from build123d import *

# Parameters (mm, degrees)
SALIENTE_EXTRUIR1_DEPTH = 49
CORTAR_EXTRUIR1_DEPTH   = 70.738798384
SALIENTE_EXTRUIR3_DEPTH = 10
CROQUIS8_W              = 12
CROQUIS8_H              = 10
CORTAR_EXTRUIR2_DEPTH   = 6.5
CROQUIS9_W              = 20
CROQUIS9_H              = 12
SALIENTE_EXTRUIR4_DEPTH = 1.5
CROQUIS10_W             = 49
CROQUIS10_H             = 45
CORTAR_EXTRUIR6_DEPTH   = 16
CROQUIS13_W             = 2
CROQUIS13_H             = 10
CORTAR_EXTRUIR7_DEPTH   = 64.131209746


with BuildPart() as part:
    # Croquis1 → Saliente-Extruir1 (new body)
    with BuildSketch(Plane.XY):
        Polygon((-3.5, 49.5), (-3.5, 0), (0, 0), (0, 41.994225778), align=None)
    extrude(amount=SALIENTE_EXTRUIR1_DEPTH)

    # Croquis2 → Cortar-Extruir1 (cut, through all)
    with BuildSketch(Plane(origin=(0, 0, 0), x_dir=(0, 0, -1), z_dir=(1, 0, 0))):
        Polygon((-49, 0), (0, 0), (0, 28.994225778), (-14.5, 28.994225778), (-14.5, 4.5), (-34.5, 4.5), (-34.5, 28.994225778), (-49, 28.994225778), align=None)
    extrude(amount=-CORTAR_EXTRUIR1_DEPTH, mode=Mode.SUBTRACT)

    # Croquis4 → Saliente-Extruir3 (add)
    with BuildSketch(Plane.XZ.offset(-28.994225778)):
        Polygon((0, 49), (20.5, 49), (20.5, 0), (0, 0), (0, 1.5), (12.5, 1.5), (12.5, 47.5), (0, 47.5), align=None)
    extrude(amount=-SALIENTE_EXTRUIR3_DEPTH)

    # Croquis8 → Cortar-Extruir2 (cut)
    with BuildSketch(Plane(origin=(20.5, 0, 0), x_dir=(0, 0, -1), z_dir=(1, 0, 0))):
        with Locations((-24.5, 33.994225778)):
            Rectangle(CROQUIS8_W, CROQUIS8_H)
        Polygon((-48, 38.994225778), (-44.360297657, 28.994225778), (-31.590164388, 28.994225778), (-35.22986673, 38.994225778), align=None)
        Polygon((-17.409835612, 28.994225778), (-4.639702343, 28.994225778), (-1, 38.994225778), (-13.77013327, 38.994225778), align=None)
    extrude(amount=-CORTAR_EXTRUIR2_DEPTH, mode=Mode.SUBTRACT)

    # Croquis9 → Saliente-Extruir4 (add)
    with BuildSketch(Plane(origin=(0, 0, 0), x_dir=(0, 0, -1), z_dir=(1, 0, 0))):
        with Locations((-24.5, 10.5)):
            Rectangle(CROQUIS9_W, CROQUIS9_H)
    extrude(amount=SALIENTE_EXTRUIR4_DEPTH)

    # Croquis10 → Cortar-Extruir6 (cut)
    with BuildSketch(Plane.ZY.offset(3.5)):
        with Locations((24.5, 27)):
            Rectangle(CROQUIS10_W, CROQUIS10_H)
    extrude(amount=-CORTAR_EXTRUIR6_DEPTH, mode=Mode.SUBTRACT)

    # Croquis13 → Cortar-Extruir7 (cut, through all)
    with BuildSketch(Plane(origin=(20.5, 0, 0), x_dir=(0, 0, -1), z_dir=(1, 0, 0))):
        with Locations((-48, 33.994225778)):
            Rectangle(CROQUIS13_W, CROQUIS13_H)
        with Locations((-1, 33.994225778)):
            Rectangle(CROQUIS13_W, CROQUIS13_H)
    extrude(amount=-CORTAR_EXTRUIR7_DEPTH, mode=Mode.SUBTRACT)


solid = part.part
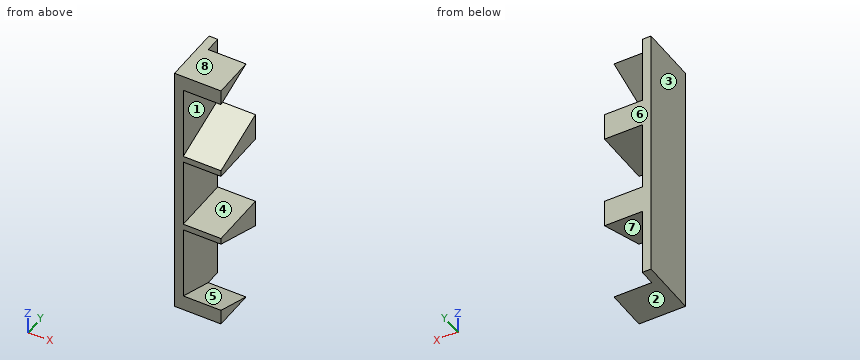
Geometry: final body of the model. Coordinates: model frame, mm. Face numbers are marked on the shaded views. A direction names the side the tool comes from. Round coordinates to 2 decimals unless told otherwise and drop trailing zeros. Loops run counter-clockwise (first coordinate to the right, second up) from the corner with the lowest first, then second, coordinate; pieces in that order, holes last.
Q1. Section D-D on y = 30.25. Return loops of the section in (x, z).
Q2. Access query for the marked faces 4, 5, 6, 7 and 8. Directions: +Z, -Z, +X, -X, +Y, -Y. A direction counts if a zero-diameter tool reaches every point of the face in a straight line with its end or side. Return the directions, or none.
Q3. Pull-direction query (Z, two-part tool) for the marked faces 1, 2 and 3; classes: released by +Z, released by -Z, zero draft, split by the parting line, or undercut.
Q4. Section A-A on x = 16.5. Return loops of the section in (y, z), plus the area to 3 significant figures.
Q5. Section B-B on y = 38. Return loops of the section in (x, z), plus the area to 3 significant figures.
Q6. Section C-C on z = 43.5. Return loops of the section in (x, y), plus the area to 3 significant figures.
Q7. Material intervals for L1, parallel to Z at x = 19.75, y = 30; L2, parallel to Z at x = 18.25, y = 32.75; L3, parallel to X at y = 32.75, z = 20.5, sorted ascending.
Q8. Pin query (flat end, axial travel): P1, Ø3, axis at y = 33.5, z = 25.5, coming from the +X side. Return the tip coordinate at first contact, or that it passes through.
Evaluation:
1. outline: (12.5, 2) - (20.5, 2) - (20.5, 4.18) - (14, 4.18) - (14, 16.95) - (20.5, 16.95) - (20.5, 18.5) - (14, 18.5) - (14, 30.5) - (20.5, 30.5) - (20.5, 32.05) - (14, 32.05) - (14, 44.82) - (20.5, 44.82) - (20.5, 47) - (12.5, 47) - close
2. face 4: +X, +Y, -Y
2. face 5: +X, +Y
2. face 6: +Z, -Z, +X, -X, +Y
2. face 7: +X, -Y
2. face 8: +Z, +X, -X, +Y, -Y
3. face 1: undercut
3. face 2: released by -Z
3. face 3: zero draft
4. outline: (28.99, 2) - (36.25, 2) - (28.99, 4.64) - close; (28.99, 17.41) - (38.99, 13.77) - (38.99, 18.5) - (28.99, 18.5) - close; (28.99, 30.5) - (38.99, 30.5) - (38.99, 35.23) - (28.99, 31.59) - close; (28.99, 44.36) - (36.25, 47) - (28.99, 47) - close
4. area: 77.3 mm2
5. outline: (12.5, 2) - (14, 2) - (14, 14.13) - (20.5, 14.13) - (20.5, 18.5) - (14, 18.5) - (14, 30.5) - (20.5, 30.5) - (20.5, 34.87) - (14, 34.87) - (14, 47) - (12.5, 47) - close
5. area: 124 mm2
6. outline: (12.5, 28.99) - (14, 28.99) - (14, 38.99) - (12.5, 38.99) - close
6. area: 15.0 mm2
7. L1: z = 2 to 4.27, 17.04 to 18.5, 30.5 to 31.96, 44.73 to 47
7. L2: z = 2 to 3.27, 16.04 to 18.5, 30.5 to 32.96, 45.73 to 47
7. L3: x = 12.5 to 14
8. P1: stops at x = 14
